Verification items for this drawing (mm, ordinates from the low corner). Give positions to 0.01 mm unless a question says otherwise; leave off trailing zeros. Loops run counter-clockwise (first coordinate to the right, second up) from the corner with the lowest first, then second, coordinate; pieces in that order, holes last. Notation, with made-up numbers: (-24.75, 36) -> (27.25, 36) arc R27 ccw to (27.25, 74) -> close; hole circle Ø7 at (45, 77). An arc over 180 degrees is marked (long way). Use one line per item in the form item = value. Start each with the question number.
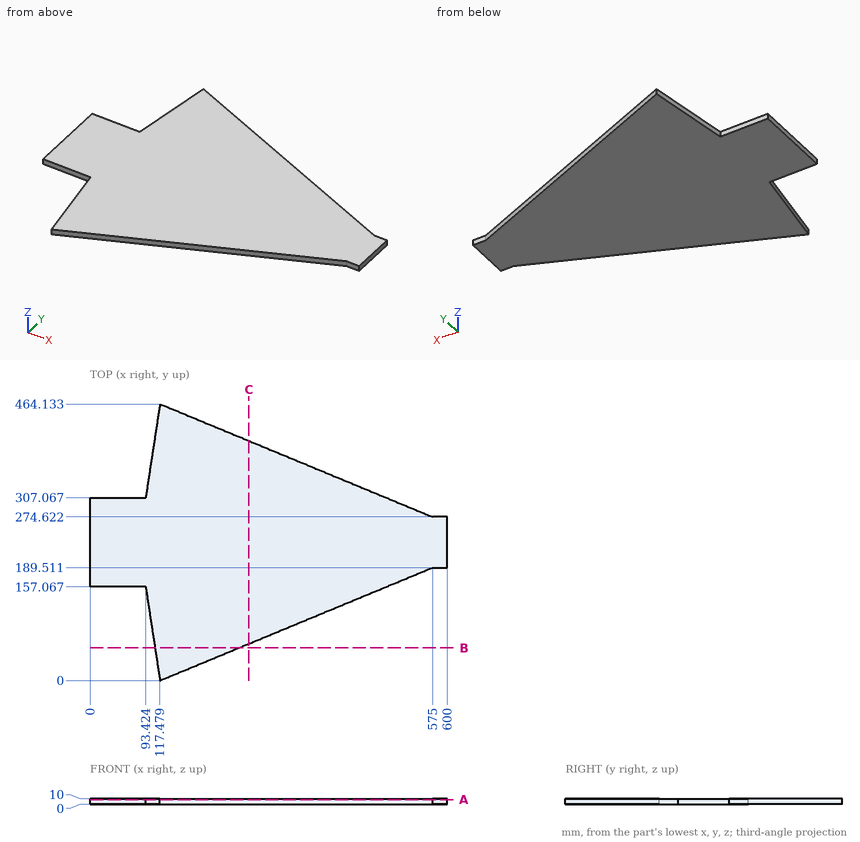
Item 1: Sectioned sample at B-B, the plane y = 55. Enter the section's corners in (x, z) (1 decimal), and give its area (3 significant figures).
Item 2: Sectioned sample at A-A, the plane z = 8.25. Enter the section's corners in (x, y) (1 decimal).
Item 3: Material ranges on line 1 (Y direction, x = 28, z = 3.5); line 2 (Y direction, x = 284, z = 8.5) (1 decimal); line 3 (X direction, y = 333, z = 5) (1 decimal), recorded low to high.
Item 4: Sectioned sample at C-C, the plane x = 266.5. Enter the section's corners in (y, z).
Item 5: Gauge pin test, flat ends, axial feed: pin 1 Ø4 at (x, z) = (488.5, 1.5) entering from +Y; pin 2 Ø3 at (x, z) = (589, 4) entering from -Y; pin 3 Ø1.5 at (y, z) = (374, 3.5) entering from +X. Record the tip position at first contact, or that the pin passes through.
Outcome:
q1.outline = (109.1, 0) -> (250.3, 0) -> (250.3, 10) -> (109.1, 10) -> close
q1.area = 1,410 mm^2
q2.outline = (0, 157.1) -> (93.4, 157.1) -> (117.5, 0) -> (575, 189.5) -> (600, 189.5) -> (600, 274.6) -> (575, 274.6) -> (117.5, 464.1) -> (93.4, 307.1) -> (0, 307.1) -> close
q3.line_1 = 157.07 to 307.07
q3.line_2 = 69 to 395.2
q3.line_3 = 97.4 to 434.1
q4.outline = (61.73, 0) -> (402.41, 0) -> (402.41, 10) -> (61.73, 10) -> close
q5.pin_1 = 311.28
q5.pin_2 = 189.51
q5.pin_3 = 336.89
